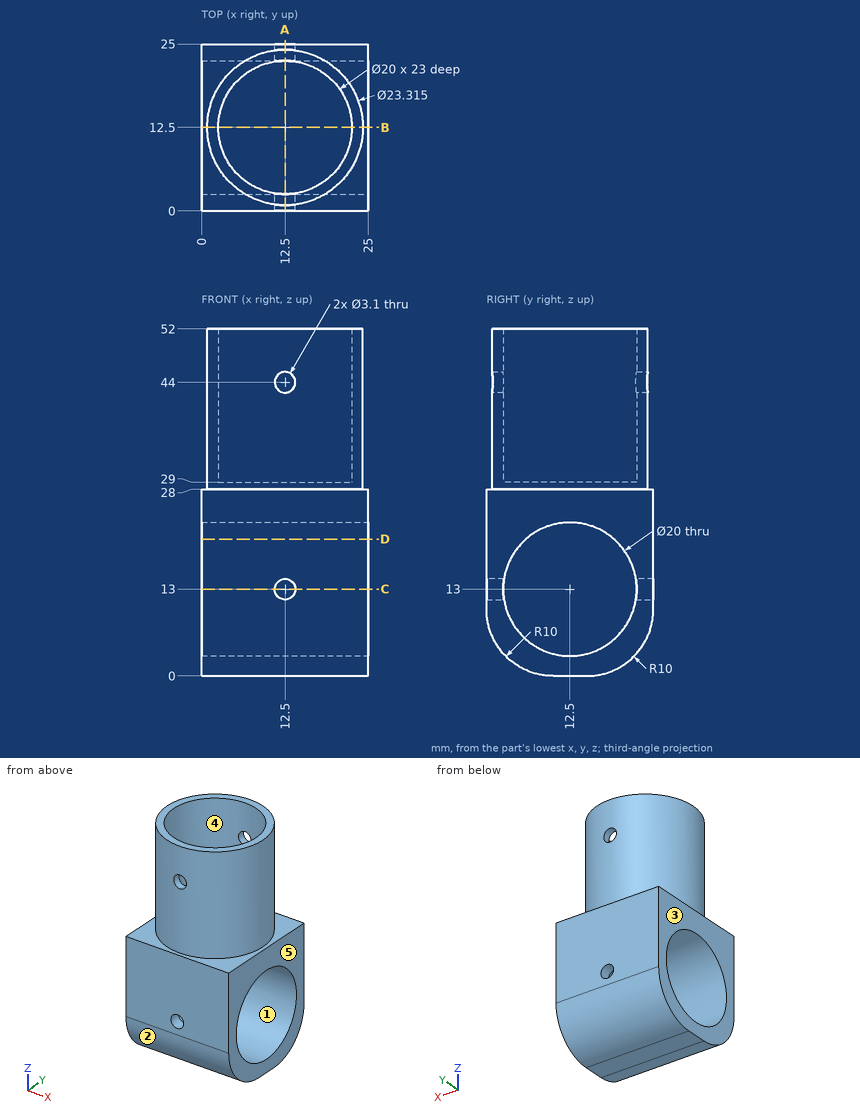
For this review, use the dimensioned drawing (mm, ordinates from the lowest corner) and the shaded views. A direction names the side the tool comes from. Coordinates: 2 decimals unless noted, no trailing zeros. Write each loop counter-clockwise with the first axis right and the second up, starting at its lowest first coordinate (ties: lowest second). Pieces come first, ordered by that corner, then holes. Notation, with made-up numbers: (51.5, 14) - (96.5, 14) arc R15 cw to (96.5, 24) - close; hole circle Ø8 at (-19, 68). An arc over 180 degrees is marked (long way). Answer in a Markdown table with one row per item. Add a question column.
Q1. To check wall thickness, follow line 1 along X through (y, z) = (1.55, 13); line 2 along X through (y, z) = (19.5, 38); line 3 along Y through (x, z) = (22.5, 6) (1 decimal). State the ranges of each line that lie inside material, in increasing order. Write a range as from..to.
Q2. Consider section A-A on x = 12.5. Give the number of separate pieces and of enclosed holes in the cut face.
Q3. Clearance check with flat-ended pins moving along their axes: pin 1 (1 mm diameter, centred on y = 11, z = 37, fed in from +X); pin 2 (2.5 mm diameter, centred on x = 12.5, z = 44, fed in from -Y); pin 3 (2 mm diameter, centred on x = 22, z = 5.5, fed in from +Y); pin 4 (3 mm diameter, centred on x = 13, y = 18.5, fed in from -Z). State where each tip first meets the part, or that it passes through.
Q4. Draft analysis for pull direction Z (two halves, no side actions). For the marked faces 1, 2 and 3, state which applies: +Z half, -Z half, draft (parallel to the pull), parting line (faces both ways), or undercut.
Q5. For the marked faces 4 and 5, list the 3-axis set-ups (+Z, -Z, +X, -X, +Y, -Y) from which the entire face can be reached by the end or side of a thin tool; tool diameter is ignored.
Q6. Consider section C-C on z = 13. Give the boundary of the cut face in (x, y), then the cut area to 4 significant figures.
Q7. Consider section D-D on z = 20.5. Give the boundary of the cut face in (x, y).
Q8. Consider section B-B on y = 12.5. Give the boundary of the cut face in (x, z).
Answers below:
| question | item | result |
|---|---|---|
| 1 | line 1 | 0..10.95, 14.05..25 |
| 1 | line 2 | 3.18..5.36, 19.64..21.82 |
| 1 | line 3 | 0.8..5.4, 19.6..24.2 |
| 2 | separate pieces | 4 |
| 2 | enclosed holes | 0 |
| 3 | pin 1 | x = 24.11 |
| 3 | pin 2 | through |
| 3 | pin 3 | y = 24.37 |
| 3 | pin 4 | z = 0.2 |
| 4 | face 1 | undercut |
| 4 | face 2 | -Z half |
| 4 | face 3 | draft |
| 5 | face 4 | +Z |
| 5 | face 5 | +Z, -Z, +X, +Y, -Y |
| 6 | outline | (0, 0) - (10.95, 0) - (10.95, 2.5) - (0, 2.5) - close; (0, 22.5) - (10.95, 22.5) - (10.95, 25) - (0, 25) - close; (14.05, 0) - (25, 0) - (25, 2.5) - (14.05, 2.5) - close; (14.05, 22.5) - (25, 22.5) - (25, 25) - (14.05, 25) - close |
| 6 | area | 109.5 mm² |
| 7 | outline | (0, 0) - (25, 0) - (25, 5.89) - (0, 5.89) - close; (0, 19.11) - (25, 19.11) - (25, 25) - (0, 25) - close |
| 8 | outline | (0, 0) - (25, 0) - (25, 3) - (0, 3) - close; (0, 23) - (25, 23) - (25, 28) - (24.16, 28) - (24.16, 52) - (22.5, 52) - (22.5, 29) - (2.5, 29) - (2.5, 52) - (0.84, 52) - (0.84, 28) - (0, 28) - close |
